Check sheet for the drawn part. Datum: minimum x, y, z corner. Units: mm. Give positions to 0.01 mm unless a question says otherwise; leave off trailing zeros. Write each loop counter-clockwise with the first axis right and the second up, starting at its lowest first coordinate (ties: lowest second). Pieces come first, ordered by that corner, then holes. Notation, with made-up numbers: (40, -23.5) -> (90, -23.5) arc R13 cw to (90, -11.5) -> close; hole circle Ø9 at (37, 75). An arc over 180 degrees is marked (long way). Write item = value, one per line. Start each with the question number.
1. Thickness scan on line 1 along X through (y, z) = (5, 148); line 2 along Z through (x, y) = (111.5, 6.25). Record the ranges inside material, lowest first.
2. Cross-section at D-D, the plane z = 135. Record the cut outline in (x, y) (1 decimal), plus the area to 3 significant figures.
3. Cross-section at A-A, the plane z = 43. Record the cut outline in (x, y), plus the area to 3 significant figures.
4. Depth check by flat-ended pin: P1, Ø1, axis at y = 5.5, z = 129.5, coming from the -X side; P2, Ø10.5, axis at x = 22, z = 106, coming from the -Y side. Enter the tip coordinate at first touch or a pass-through.
5. Cross-section at B-B, the plane x = 22. Record the cut outline in (y, z), plus the area to 3 significant figures.
6. Cross-section at C-C, the plane z = 106. Record the cut outline in (x, y).
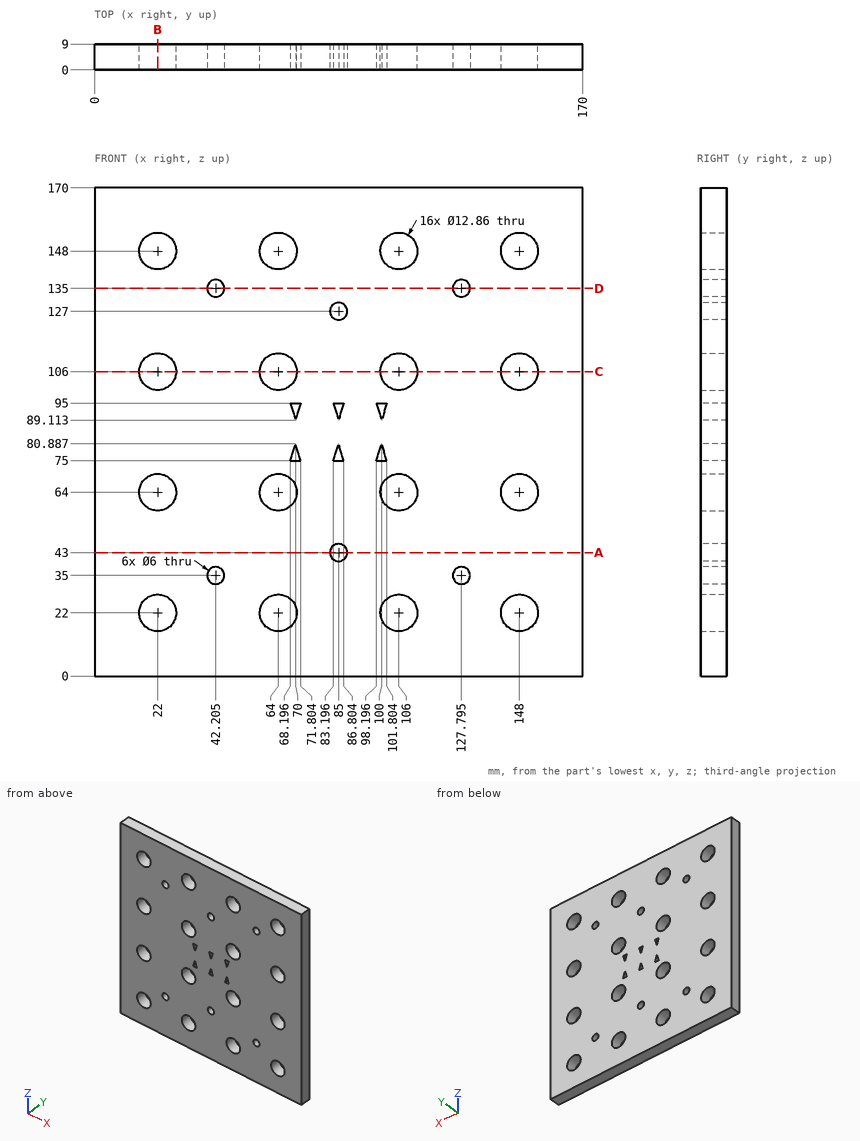
Answers:
q1.line_1 = 0 to 15.57, 28.43 to 57.57, 70.43 to 99.57, 112.43 to 141.57, 154.43 to 170
q1.line_2 = 0 to 18.67, 25.33 to 60.67, 67.33 to 102.67, 109.33 to 144.67, 151.33 to 170
q2.outline = (0, 0) -> (39.2, 0) -> (39.2, 9) -> (0, 9) -> close; (45.2, 0) -> (124.8, 0) -> (124.8, 9) -> (45.2, 9) -> close; (130.8, 0) -> (170, 0) -> (170, 9) -> (130.8, 9) -> close
q2.area = 1,420 mm^2
q3.outline = (0, 0) -> (82, 0) -> (82, 9) -> (0, 9) -> close; (88, 0) -> (170, 0) -> (170, 9) -> (88, 9) -> close
q3.area = 1,480 mm^2
q4.P1 = 0
q4.P2 = through
q5.outline = (0, 0) -> (9, 0) -> (9, 15.57) -> (0, 15.57) -> close; (0, 28.43) -> (9, 28.43) -> (9, 57.57) -> (0, 57.57) -> close; (0, 70.43) -> (9, 70.43) -> (9, 99.57) -> (0, 99.57) -> close; (0, 112.43) -> (9, 112.43) -> (9, 141.57) -> (0, 141.57) -> close; (0, 154.43) -> (9, 154.43) -> (9, 170) -> (0, 170) -> close
q5.area = 1,070 mm^2
q6.outline = (0, 0) -> (15.57, 0) -> (15.57, 9) -> (0, 9) -> close; (28.43, 0) -> (57.57, 0) -> (57.57, 9) -> (28.43, 9) -> close; (70.43, 0) -> (99.57, 0) -> (99.57, 9) -> (70.43, 9) -> close; (112.43, 0) -> (141.57, 0) -> (141.57, 9) -> (112.43, 9) -> close; (154.43, 0) -> (170, 0) -> (170, 9) -> (154.43, 9) -> close
